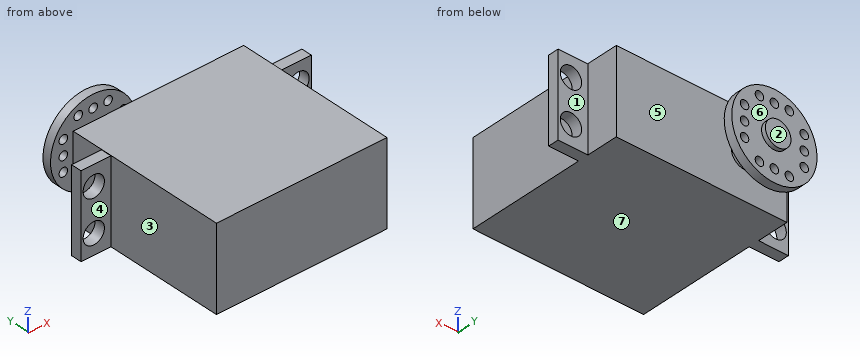
from build123d import *

# Parameters (mm, degrees)
SKETCH_1_W      = 40
SKETCH_1_H      = 38
EXTRUDE_1_DEPTH = 19.5
EXTRUDE_START   = -10
SKETCH_2_W      = 7
SKETCH_2_H      = 19.419635957
SKETCH_2_R      = 2.5
EXTRUDE_2_DEPTH = 2.5
SKETCH_3_R      = 3
EXTRUDE_3_DEPTH = 6
SKETCH_4_R      = 10
SKETCH_4_R_2    = 1
EXTRUDE_4_DEPTH = 2
SKETCH_5_R      = 3
EXTRUDE_5_DEPTH = 1


with BuildPart() as part:
    # 草图1 → 凸台-拉伸1 (new body)
    with BuildSketch(Plane.XY):
        with Locations((20, 19)):
            Rectangle(SKETCH_1_W, SKETCH_1_H)
    extrude(amount=EXTRUDE_1_DEPTH)

    # 草图2 → 凸台-拉伸2 (add)
    # profile 1 of 2: a face of its own
    with BuildSketch(Plane(origin=(0, 38, 0), x_dir=(1, 0, 0), z_dir=(0, 1, 0)).offset(EXTRUDE_START)):
        with Locations((43.5, -9.709817979)):
            Rectangle(SKETCH_2_W, SKETCH_2_H)
        with Locations(Location((44, -4.709817978, 0), (0, 0, 270))):
            Circle(SKETCH_2_R, mode=Mode.SUBTRACT)
        with Locations(Location((44, -14.709817978, 0), (0, 0, 90))):
            Circle(SKETCH_2_R, mode=Mode.SUBTRACT)
    # profile 2 of 2: a face of its own
    with BuildSketch(Plane(origin=(0, 38, 0), x_dir=(1, 0, 0), z_dir=(0, 1, 0)).offset(EXTRUDE_START)):
        with Locations((-3.5, -9.709817979)):
            Rectangle(SKETCH_2_W, SKETCH_2_H)
        with Locations(Location((-4, -14.709817978, 0), (0, 0, 270))):
            Circle(SKETCH_2_R, mode=Mode.SUBTRACT)
        with Locations(Location((-4, -4.709817978, 0), (0, 0, 90))):
            Circle(SKETCH_2_R, mode=Mode.SUBTRACT)
    extrude(amount=EXTRUDE_2_DEPTH)

    # 草图3 → 凸台-拉伸3 (add)
    with BuildSketch(Plane(origin=(0, 38, 0), x_dir=(1, 0, 0), z_dir=(0, 1, 0))):
        with Locations(Location((10, -9.75, 0), (0, 0, 90))):
            Circle(SKETCH_3_R)
    extrude(amount=EXTRUDE_3_DEPTH)

    # 草图4 → 凸台-拉伸4 (add)
    with BuildSketch(Plane(origin=(0, 44, 0), x_dir=(1, 0, 0), z_dir=(0, 1, 0))):
        with Locations(Location((10, -9.75, 0), (0, 0, 270))):
            Circle(SKETCH_4_R)
        with Locations(Location((10, -2.75, 0), (0, 0, 270))):
            Circle(SKETCH_4_R_2, mode=Mode.SUBTRACT)
        with Locations(Location((13.5, -2.75, 0), (0, 0, 270))):
            Circle(SKETCH_4_R_2, mode=Mode.SUBTRACT)
        with Locations(Location((6.5, -2.75, 0), (0, 0, 270))):
            Circle(SKETCH_4_R_2, mode=Mode.SUBTRACT)
        with Locations(Location((6.5, -16.75, 0), (0, 0, 90))):
            Circle(SKETCH_4_R_2, mode=Mode.SUBTRACT)
        with Locations(Location((13.5, -16.75, 0), (0, 0, 90))):
            Circle(SKETCH_4_R_2, mode=Mode.SUBTRACT)
        with Locations(Location((10, -16.75, 0), (0, 0, 90))):
            Circle(SKETCH_4_R_2, mode=Mode.SUBTRACT)
        with Locations(Location((3, -13.25, 0), (0, 0, 270))):
            Circle(SKETCH_4_R_2, mode=Mode.SUBTRACT)
        with Locations(Location((3, -9.75, 0), (0, 0, 270))):
            Circle(SKETCH_4_R_2, mode=Mode.SUBTRACT)
        with Locations(Location((3, -6.25, 0), (0, 0, 270))):
            Circle(SKETCH_4_R_2, mode=Mode.SUBTRACT)
        with Locations(Location((17, -6.25, 0), (0, 0, 90))):
            Circle(SKETCH_4_R_2, mode=Mode.SUBTRACT)
        with Locations(Location((17, -9.75, 0), (0, 0, 90))):
            Circle(SKETCH_4_R_2, mode=Mode.SUBTRACT)
        with Locations(Location((17, -13.25, 0), (0, 0, 90))):
            Circle(SKETCH_4_R_2, mode=Mode.SUBTRACT)
    extrude(amount=EXTRUDE_4_DEPTH)

    # 草图5 → 凸台-拉伸5 (add)
    with BuildSketch(Plane(origin=(0, 46, 0), x_dir=(1, 0, 0), z_dir=(0, 1, 0))):
        with Locations(Location((10, -9.75, 0), (0, 0, 90))):
            Circle(SKETCH_5_R)
    extrude(amount=EXTRUDE_5_DEPTH)


solid = part.part
Here's how the part is built. I have some questions about the finished solid (model axes, mm). Face numbers are marked on the shaded views. A direction names the side the tool comes from. Coordinates: 2 decimals unless noted, no trailing zeros. Loops run counter-clockwise (first coordinate to the right, second up) from the corner with the lowest first, then second, coordinate; pieces in that order, holes last.
1. I need wall thicknesses on L1, parallel to Y at x = 3, z = 8; L2, parallel to X at y = 44.95, z = 13.25; L3, parallel to X at y = 44.7, z = 16.75. Which ranges of each line are inside material? Lowest first, please.
2. For P1, Ø2, axis at x = 43, y = 29, coming from the +Z side; P2, Ø3, axis at x = 34.5, z = 6.5, coming from the +Y side; P3, Ø7.5, axis at x = 42, z = 7.5, coming from the -Y side; P4, Ø1.5, axis at x = 41.5, z = 14.5, coming from the -Y side, each with a flat end and sliding along its axis, tell me the tip position at first contact or that it passes through.
3. For the marked faces 1, 2 and 3, which set-ups out of +Z, -Z, +X, -X, +Y, -Y let a thin tool reach every point of the face, with its end or its side?
4. Imagine slicing it at D-D, the plane y = 41.5. Please give me the cut outline in (x, z).
5. Imagine slicing it at B-B, the plane x = 10. Please give me the cut outline in (y, z), and give its area (3 significant figures).
6. Imagine slicing it at C-C, the plane x = 3. Please give me the cut outline in (y, z), and give its area (3 significant figures).
7. Imagine slicing it at A-A, the plane z = 9.75. Count the separate pieces of the cut face and the enclosed holes in it, and give its area (3 significant figures).
8. If we mould it in two halves opening along Y, with no side actions, what happens to the marked faces 4, 5, 6 and 7? For each: pulls with the +Y half, pulls with the -Y half, needs draft (parallel to the pull), parting line crosses it, or undercut.
Taken from the geometry:
1. L1: y = 0 to 38, 44 to 46
1. L2: x = 0.63 to 2, 4 to 16, 18 to 19.37
1. L3: x = 2.86 to 5.5, 7.5 to 9, 11 to 12.5, 14.5 to 17.14
2. P1: stops at z = 19.42
2. P2: stops at y = 38
2. P3: stops at y = 0
2. P4: stops at y = 28
3. face 1: +Z, -Z, +X, +Y
3. face 2: +Z, -Z, +X, -X, +Y
3. face 3: +Z, -Z, -X
4. outline: circle Ø6 at (10, 9.75)
5. outline: (0, 0) - (38, 0) - (38, 6.75) - (44, 6.75) - (44, 3.75) - (46, 3.75) - (46, 6.75) - (47, 6.75) - (47, 12.75) - (46, 12.75) - (46, 15.75) - (44, 15.75) - (44, 12.75) - (38, 12.75) - (38, 19.5) - (0, 19.5) - close; (44, -0.25) - (46, -0.25) - (46, 1.75) - (44, 1.75) - close; (44, 17.75) - (46, 17.75) - (46, 19.75) - (44, 19.75) - close
5. area: 815 mm2
6. outline: (0, 0) - (38, 0) - (38, 19.5) - (0, 19.5) - close; (44, 2.61) - (46, 2.61) - (46, 5.25) - (44, 5.25) - close; (44, 7.25) - (46, 7.25) - (46, 8.75) - (44, 8.75) - close; (44, 10.75) - (46, 10.75) - (46, 12.25) - (44, 12.25) - close; (44, 14.25) - (46, 14.25) - (46, 16.89) - (44, 16.89) - close
6. area: 758 mm2
7. separate pieces: 3
7. enclosed holes: 0
7. area: 1,630 mm2
8. face 4: pulls with the -Y half
8. face 5: undercut
8. face 6: pulls with the +Y half
8. face 7: needs draft
